Check sheet for the modelled part. Datum: model origin and axes. Units: mm. Coordinates: 2 decimals unless noted, no trailing zeros. Loops run counter-clockwise (first coordinate to the right, second up) from the corner with the lowest first, then second, coordinate; pieces in that order, holes last. Notation, with made-up numbers: (-31, 88.5) -> (-21, 88.5) arc R16 ccw to (-21, 100.5) -> close; hole circle Ø4 at (0, -1). An arc over 180 degrees is marked (long way). Use CSV: the item, a comma, the result in double quotes. Start each with the question number.
1. Sectioned sample at B-B, the plane y = 228.5. Record the cut outline in (x, z).
2. Thickness scan on L1, parallel to X at y = 285, z = 3.1; L2, parallel to X at y = 328, z = 2.35; L3, parallel to Y at x = 292, z = 2.6 (3 decimals). Record the ranges inside material, lowest first.
3. Sectioned sample at A-A, the plane x = 268. Record the cut outline in (y, z).
4. Gauge pin test, flat ends, axial feed: pin 1 (3.5 mm diameter, centred on x = 236.5, z = 3.5, fed in from -Y); pin 2 (1.6 mm diameter, centred on x = 313, z = 3, fed in from +Y). Record the tip position at first contact, or that the pin passes through.
5. Sectioned sample at C-C, the plane z = 3.2. Count the separate pieces of the cut face and the enclosed holes in it, and give its area (3 significant figures).
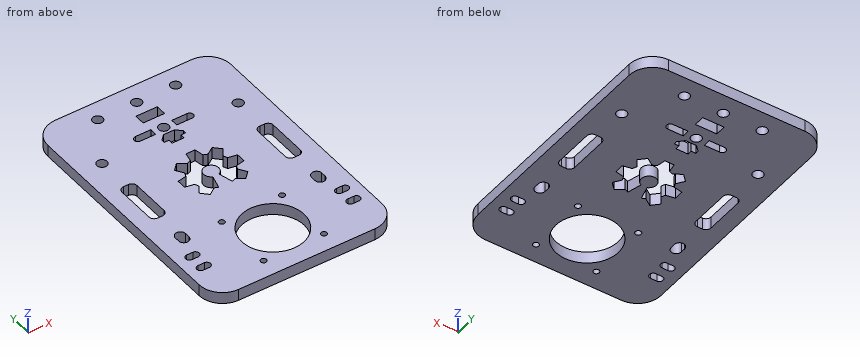
```python
from build123d import *

# Parameters (mm, degrees)
CROQUIS1_R              = 1.5
CROQUIS1_R_2            = 16
CROQUIS1_R_3            = 2.6
CROQUIS1_W              = 11
CROQUIS1_H              = 5.4
SALIENTE_EXTRUIR1_DEPTH = 6


with BuildPart() as part:
    # Croquis1 → Saliente-Extruir1 (new body)
    with BuildSketch(Plane.XY):
        with BuildLine():
            Line((240.259705315, 349.798608336), (310.25970522, 349.798608336))
            ThreePointArc((310.25970522, 349.798608336), (318.706095722, 346.299998838), (322.204705221, 337.853608336))
            Line((322.204705221, 337.853608336), (322.20470522, 226.043602373))
            ThreePointArc((322.20470522, 226.043602373), (318.706095721, 217.597211872), (310.25970522, 214.098602373))
            Line((310.25970522, 214.098602373), (240.259705314, 214.098602373))
            ThreePointArc((240.259705314, 214.098602373), (231.813314813, 217.597211873), (228.314705315, 226.043602374))
            Line((228.314705315, 226.043602374), (228.314705315, 337.853608336))
            ThreePointArc((228.314705315, 337.853608336), (231.813314814, 346.299998837), (240.259705315, 349.798608336))
        make_face()
        with Locations((259.759705267, 223.648603564)):
            Circle(CROQUIS1_R, mode=Mode.SUBTRACT)
        with Locations((290.759705267, 223.648603373)):
            Circle(CROQUIS1_R, mode=Mode.SUBTRACT)
        with Locations((290.759705459, 254.648603373)):
            Circle(CROQUIS1_R, mode=Mode.SUBTRACT)
        with Locations((259.759705459, 254.648603564)):
            Circle(CROQUIS1_R, mode=Mode.SUBTRACT)
        with Locations((275.259705363, 239.148602396)):
            Circle(CROQUIS1_R_2, mode=Mode.SUBTRACT)
        with Locations((310.25970522, 315.148608341)):
            Circle(CROQUIS1_R_3, mode=Mode.SUBTRACT)
        with Locations((240.259705315, 315.148608341)):
            Circle(CROQUIS1_R_3, mode=Mode.SUBTRACT)
        with Locations((275.259705268, 319.839051264)):
            Circle(CROQUIS1_R_3, mode=Mode.SUBTRACT)
        with Locations((295.259705059, 339.839051264)):
            Circle(CROQUIS1_R_3, mode=Mode.SUBTRACT)
        with Locations((275.259705268, 339.839051072)):
            Circle(CROQUIS1_R_3, mode=Mode.SUBTRACT)
        with Locations((255.259705059, 339.839051264)):
            Circle(CROQUIS1_R_3, mode=Mode.SUBTRACT)
        with BuildLine():
            Line((312.85970522, 254.648608341), (312.85970522, 257.148608341))
            ThreePointArc((312.85970522, 257.148608341), (310.25970522, 259.748608341), (307.65970522, 257.148608341))
            Line((307.65970522, 257.148608341), (307.65970522, 254.648608341))
            ThreePointArc((307.65970522, 254.648608341), (310.25970522, 252.048608341), (312.85970522, 254.648608341))
        make_face(mode=Mode.SUBTRACT)
        with BuildLine():
            Line((312.119953493, 241.436102396), (315.334279571, 241.436102396))
            ThreePointArc((315.334279571, 241.436102396), (317.221779571, 243.323602396), (315.334279571, 245.211102396))
            Line((315.334279571, 245.211102396), (312.119953493, 245.211102396))
            ThreePointArc((312.119953493, 245.211102396), (310.232453493, 243.323602396), (312.119953493, 241.436102396))
        make_face(mode=Mode.SUBTRACT)
        with BuildLine():
            Line((315.334279571, 233.011268799), (312.119953493, 233.011268799))
            ThreePointArc((312.119953493, 233.011268799), (310.232453493, 234.898768799), (312.119953493, 236.786268799))
            Line((312.119953493, 236.786268799), (315.334279571, 236.786268799))
            ThreePointArc((315.334279571, 236.786268799), (317.221779571, 234.898768799), (315.334279571, 233.011268799))
        make_face(mode=Mode.SUBTRACT)
        with BuildLine():
            Line((238.399457042, 233.011268799), (235.185130964, 233.011268799))
            ThreePointArc((235.185130964, 233.011268799), (233.297630964, 234.898768799), (235.185130964, 236.786268799))
            Line((235.185130964, 236.786268799), (238.399457042, 236.786268799))
            ThreePointArc((238.399457042, 236.786268799), (240.286957042, 234.898768799), (238.399457042, 233.011268799))
        make_face(mode=Mode.SUBTRACT)
        with BuildLine():
            Line((238.399457042, 241.436102396), (235.185130964, 241.436102396))
            ThreePointArc((235.185130964, 241.436102396), (233.297630964, 243.323602396), (235.185130964, 245.211102396))
            Line((235.185130964, 245.211102396), (238.399457042, 245.211102396))
            ThreePointArc((238.399457042, 245.211102396), (240.286957042, 243.323602396), (238.399457042, 241.436102396))
        make_face(mode=Mode.SUBTRACT)
        with BuildLine():
            Line((237.659705315, 254.648608341), (237.659705315, 257.148608341))
            ThreePointArc((237.659705315, 257.148608341), (240.259705315, 259.748608341), (242.859705315, 257.148608341))
            Line((242.859705315, 257.148608341), (242.859705315, 254.648608341))
            ThreePointArc((242.859705315, 254.648608341), (240.259705315, 252.048608341), (237.659705315, 254.648608341))
        make_face(mode=Mode.SUBTRACT)
        with BuildLine():
            Line((264.517482129, 281.575286085), (259.966113425, 282.436756346))
            Line((259.966113425, 282.436756346), (259.966113425, 287.16046109))
            Line((259.966113425, 287.16046109), (264.517482129, 288.021931352))
            Line((264.517482129, 288.021931352), (265.38457315, 290.115274253))
            Line((265.38457315, 290.115274253), (262.775420938, 293.942729391))
            Line((262.775420938, 293.942729391), (266.115584595, 297.282893048))
            Line((266.115584595, 297.282893048), (269.943039733, 294.673740836))
            Line((269.943039733, 294.673740836), (272.036382634, 295.540831857))
            Line((272.036382634, 295.540831857), (272.897852896, 300.092200561))
            Line((272.897852896, 300.092200561), (277.621557639, 300.092200561))
            Line((277.621557639, 300.092200561), (278.483027901, 295.540831857))
            Line((278.483027901, 295.540831857), (280.576370802, 294.673740836))
            Line((280.576370802, 294.673740836), (284.40382594, 297.282893048))
            Line((284.40382594, 297.282893048), (287.743989597, 293.942729391))
            Line((287.743989597, 293.942729391), (285.134837385, 290.115274253))
            Line((285.134837385, 290.115274253), (286.001928406, 288.021931352))
            Line((286.001928406, 288.021931352), (290.55329711, 287.16046109))
            Line((290.55329711, 287.16046109), (290.55329711, 282.436756346))
            Line((290.55329711, 282.436756346), (286.001928406, 281.575286085))
            Line((286.001928406, 281.575286085), (285.134837385, 279.481943184))
            Line((285.134837385, 279.481943184), (287.743989597, 275.654488046))
            Line((287.743989597, 275.654488046), (284.40382594, 272.314324389))
            Line((284.40382594, 272.314324389), (280.576370802, 274.923476601))
            Line((280.576370802, 274.923476601), (278.743688474, 274.164354725))
            Line((278.743688474, 274.164354725), (276.840273676, 281.267995461))
            ThreePointArc((276.840273676, 281.267995461), (275.259705267, 288.66686756), (273.679136859, 281.267995461))
            Line((273.679136859, 281.267995461), (271.775722061, 274.164354725))
            Line((271.775722061, 274.164354725), (269.943039733, 274.923476601))
            Line((269.943039733, 274.923476601), (266.115584595, 272.314324389))
            Line((266.115584595, 272.314324389), (262.775420938, 275.654488046))
            Line((262.775420938, 275.654488046), (265.38457315, 279.481943184))
            Line((265.38457315, 279.481943184), (264.517482129, 281.575286085))
        make_face(mode=Mode.SUBTRACT)
        with BuildLine():
            Line((244.109705315, 274.798608718), (244.109705315, 294.798608718))
            ThreePointArc((244.109705315, 294.798608718), (243.348182946, 296.63708635), (241.509705315, 297.398608718))
            Line((241.509705315, 297.398608718), (239.009705315, 297.398608718))
            ThreePointArc((239.009705315, 297.398608718), (237.171227684, 296.63708635), (236.409705315, 294.798608718))
            Line((236.409705315, 294.798608718), (236.409705315, 274.798608718))
            ThreePointArc((236.409705315, 274.798608718), (237.171227684, 272.960131087), (239.009705315, 272.198608718))
            Line((239.009705315, 272.198608718), (241.509705315, 272.198608718))
            ThreePointArc((241.509705315, 272.198608718), (243.348182946, 272.960131087), (244.109705315, 274.798608718))
        make_face(mode=Mode.SUBTRACT)
        with BuildLine():
            Line((314.10970522, 294.798608718), (314.10970522, 274.798608718))
            ThreePointArc((314.10970522, 274.798608718), (313.348182851, 272.960131087), (311.50970522, 272.198608718))
            Line((311.50970522, 272.198608718), (309.00970522, 272.198608718))
            ThreePointArc((309.00970522, 272.198608718), (307.171227589, 272.960131087), (306.40970522, 274.798608718))
            Line((306.40970522, 274.798608718), (306.40970522, 294.798608718))
            ThreePointArc((306.40970522, 294.798608718), (307.171227589, 296.63708635), (309.00970522, 297.398608718))
            Line((309.00970522, 297.398608718), (311.50970522, 297.398608718))
            ThreePointArc((311.50970522, 297.398608718), (313.348182851, 296.63708635), (314.10970522, 294.798608718))
        make_face(mode=Mode.SUBTRACT)
        Polygon((272.134705268, 309.294051072), (278.384705268, 309.294051072), (278.38470522, 311.598608336), (280.75970522, 311.598608336), (280.759705268, 313.278390901), (278.099045096, 315.939051072), (272.420365439, 315.939051072), (269.759705268, 313.278390901), (269.75970522, 311.598608336), (272.13470522, 311.598608336), align=None, mode=Mode.SUBTRACT)
        with BuildLine():
            Line((269.859705268, 318.001551072), (261.919333168, 318.001551072))
            ThreePointArc((261.919333168, 318.001551072), (260.081833168, 319.839051072), (261.919333168, 321.676551072))
            Line((261.919333168, 321.676551072), (269.859705268, 321.676551072))
            Line((269.859705268, 321.676551072), (269.859705268, 318.001551072))
        make_face(mode=Mode.SUBTRACT)
        with BuildLine():
            Line((288.600077367, 321.676551072), (280.659705268, 321.676551072))
            Line((280.659705268, 321.676551072), (280.659705268, 318.001551072))
            Line((280.659705268, 318.001551072), (288.600077367, 318.001551072))
            ThreePointArc((288.600077367, 318.001551072), (290.437577367, 319.839051072), (288.600077367, 321.676551072))
        make_face(mode=Mode.SUBTRACT)
        with Locations((275.259705268, 329.839051072)):
            Rectangle(CROQUIS1_W, CROQUIS1_H, mode=Mode.SUBTRACT)
    extrude(amount=SALIENTE_EXTRUIR1_DEPTH)


solid = part.part
```
Completed:
1,outline,"(228.31, 0) -> (263.32, 0) -> (263.32, 6) -> (228.31, 6) -> close; (287.2, 0) -> (322.2, 0) -> (322.2, 6) -> (287.2, 6) -> close"
2,L1,"228.31 to 236.41, 244.11 to 259.97, 271.4 to 279.12, 290.55 to 306.41, 314.11 to 322.2"
2,L2,"228.31 to 269.76, 280.76 to 322.2"
2,L3,"214.099 to 222.805, 224.492 to 253.805, 255.492 to 349.799"
3,outline,"(214.1, 0) -> (224.89, 0) -> (224.89, 6) -> (214.1, 6) -> close; (253.41, 0) -> (273.6, 0) -> (273.6, 6) -> (253.41, 6) -> close; (296, 0) -> (318, 0) -> (318, 6) -> (296, 6) -> close; (321.68, 0) -> (349.8, 0) -> (349.8, 6) -> (321.68, 6) -> close"
4,pin 1,"y = 214.27"
4,pin 2,"y = 349.64"
5,separate pieces,"1"
5,enclosed holes,"24"
5,area,"10,500 mm²"
